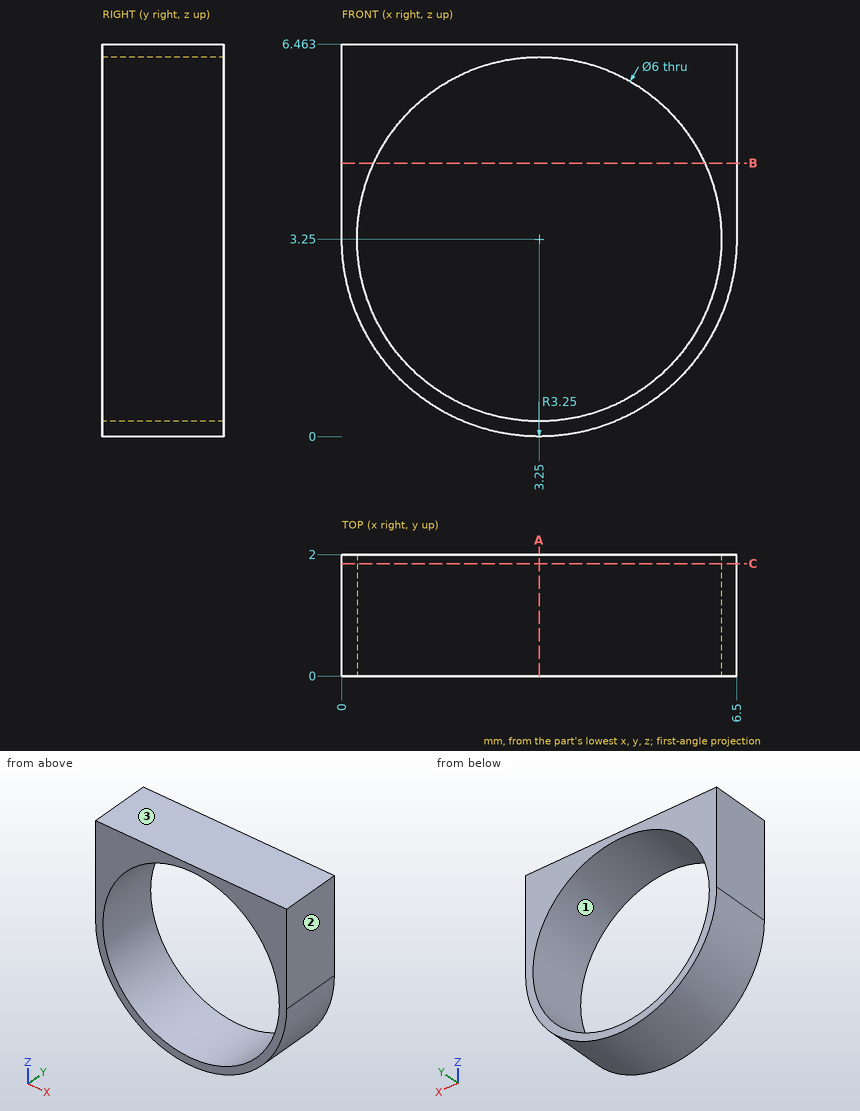
Part print with two shaded views. Sizes in mm from the minimum x, y, z corner. Coordinates: 2 decimals unless noted, no trailing zeros. Write each loop counter-clockwise with the first axis right and the second up, starting at its lowest first coordinate (ties: lowest second). Pieces come first, ordered by that corner, then holes. Notation, with made-up numbers: (-25.5, 30) - (2.5, 30) arc R17 cw to (2.5, 47) - close; hole circle Ø4 at (65, 87.5). An arc over 180 degrees is marked (long way). Use a Markdown table: item, result. Add a question column.
Item 1: Band-saw the part on C-C, the plane y = 1.85. Write the cut outline in (x, z).
Item 2: Drill centre lines: line 1 along X through (y, z) = (0.5, 3.25); line 2 along X through (y, z) = (0.8, 5.75); line 3 along Z through (x, y) = (5.25, 0.2) (1 decimal). Where is each one in solid material? Low to high.
Item 3: Band-saw the part on B-B, the plane z = 4.5. Write the cut outline in (x, y).
Item 4: Band-saw the part on A-A, the plane x = 3.25. Write the cut outline in (y, z).
Item 5: Two-plate mould, pull along Z, no slides. Class the marked faces 1, 2 and 3: pulls with the +Z half, pulls with the -Z half, needs draft (parallel to the pull), parting line crosses it, or undercut.
A:
| question | item | result |
|---|---|---|
| 1 | outline | (0, 3.25) arc R3.25 ccw to (6.5, 3.25) - (6.5, 6.46) - (0, 6.46) - close; hole circle Ø6 at (3.25, 3.25) |
| 2 | line 1 | x = 0 to 0.25, 6.25 to 6.5 |
| 2 | line 2 | x = 0 to 1.59, 4.91 to 6.5 |
| 2 | line 3 | z = 0.7 to 1, 5.5 to 6.5 |
| 3 | outline | (0, 0) - (0.52, 0) - (0.52, 2) - (0, 2) - close; (5.98, 0) - (6.5, 0) - (6.5, 2) - (5.98, 2) - close |
| 4 | outline | (0, 0) - (2, 0) - (2, 0.25) - (0, 0.25) - close; (0, 6.25) - (2, 6.25) - (2, 6.46) - (0, 6.46) - close |
| 5 | face 1 | undercut |
| 5 | face 2 | needs draft |
| 5 | face 3 | pulls with the +Z half |
